from build123d import *

# Parameters (mm, degrees)
CYLINDER011007_R     = 2.1
CYLINDER011007_DEPTH = 20
CYLINDER011006_R     = 12
CYLINDER011006_DEPTH = 2
CYLINDER011009_R     = 0.5
CYLINDER011009_DEPTH = 7
ARRAY007_COUNT       = 22
CYLINDER011005_R     = 6
CYLINDER011005_DEPTH = 7


with BuildPart() as belt_attach_insert_hole:
    # Cylinder011007 → Cylinder011007 (new body)
    with BuildSketch(Plane.XZ):
        Circle(CYLINDER011007_R)
    extrude(amount=CYLINDER011007_DEPTH)


with BuildPart() as belt_disk:
    # Cylinder011006 → Cylinder011006 (new body)
    with BuildSketch(Plane.XZ.offset(7)):
        Circle(CYLINDER011006_R)
    extrude(amount=CYLINDER011006_DEPTH)


with BuildPart() as belt_pin_array:
    # Cylinder011009 → Cylinder011009 (new body)
    with BuildSketch(Plane(origin=(6, 0, 0), x_dir=(1, 0, 0), z_dir=(0, -1, 0))):
        Circle(CYLINDER011009_R)
    extrude(amount=CYLINDER011009_DEPTH)

    # Array007: belt pin array ×22 about axis
    array007_axis = Axis((0, 0, 0), (0, 1, 0))


with BuildPart() as belt_pin_array_1:
    add(belt_pin_array.part)
    for i in range(1, ARRAY007_COUNT):
        add(belt_pin_array.part.rotate(array007_axis, i * 360 / ARRAY007_COUNT))


with BuildPart() as belt_attach_cut:
    # Cylinder011005 → Cylinder011005 (new body)
    with BuildSketch(Plane.XZ):
        Circle(CYLINDER011005_R)
    extrude(amount=CYLINDER011005_DEPTH)

    # Fusion003: union belt disk, belt pin array
    add(belt_disk.part)
    add(belt_pin_array_1.part)

    # Cut023015009007: cut belt attach insert hole
    add(belt_attach_insert_hole.part, mode=Mode.SUBTRACT)


solid = belt_attach_cut.part
Geometry check sheet. Reference: the model listing, model coordinates, mm. A direction names the side the tool comes from. Coordinates: 2 decimals unless noted, no trailing zeros. Loops run counter-clockwise (first coordinate to the right, second up) from the corner with the lowest first, then second, coordinate; pieces in that order, holes last. Notation, with made-up numbers: (75, 34.25) - (123, 34.25) arc R35 cw to (123, 67.25) - close; hole circle Ø5 at (10, 77). An arc over 180 degrees is marked (long way). Use one line per item in the form item = value. Start each with the question number.
Item 1: Gauge pin test, flat ends, axial feed: pin 1 (4 mm diameter, centred on x = 0, z = 0, fed in from -Y); pin 2 (1 mm diameter, centred on x = 3.5, z = -6, fed in from +Y); pin 3 (4 mm diameter, centred on y = -5.5, z = 2.5, fed in from -X); pin 4 (5 mm diameter, centred on y = -1, z = -4.5, fed in from +X). Record the tip position at first contact, or that the pin passes through.
Item 2: Thickness scan on probe 1 along X at (y, z) = (-6, 0); probe 2 along Z at (x, y) = (0, -6.75); probe 3 along Z at (x, y) = (-2.5, -4.5). Record the ranges inside material, lowest first.
Item 3: Tool access check on faces 1 (the face through (2.003, -4.437, 0.631)), 2 (the face through (-6, -7, 3)). Record the directions out of +Z, -Z, +X, -X, +Y, -Y that give a thin tool (end or side, any length) a straight path to the whole face; none if there is none.
Item 4: Section check D-D, the plane x = -7. Enter the section's corners in (y, z), and give its area (3 significant figures).
Item 5: Section check B-B, the plane z = 0. Enter the section's corners in (x, y), and give its area (3 significant figures).
Item 6: Section check A-A, the plane x = 0. Enter the section's corners in (y, z).
Item 7: Section check C-C, the plane y = -8. Enter the section's corners in (x, z), and give its area (3 significant figures).
Item 8: Mould release check, pull along Z, two halves, no side actions. Record for faces 3 (the face through (2.5, -9, 0.2)), 4 (the face through (4.27, -3.45, 4.9)): +Z half, -Z half, draft (parallel to the pull), parting line (faces both ways), or undercut.
Computed:
q1.pin_1 = through
q1.pin_2 = -7
q1.pin_3 = -11.94
q1.pin_4 = 6.15
q2.probe_1 = -6.5 to -2.1, 2.1 to 6.5
q2.probe_2 = -6 to -2.1, 2.1 to 6
q2.probe_3 = -5.96 to 5.96
q3.face_1 = +Y, -Y
q3.face_2 = +Y
q4.outline = (-9, -9.75) - (-7, -9.75) - (-7, 9.75) - (-9, 9.75) - close
q4.area = 39.0 mm2
q5.outline = (-12, -9) - (-2.1, -9) - (-2.1, 0) - (-6.5, 0) - (-6.5, -7) - (-12, -7) - close; (2.1, -9) - (12, -9) - (12, -7) - (6.5, -7) - (6.5, 0) - (2.1, 0) - close
q5.area = 101 mm2
q6.outline = (-9, -12) - (-7, -12) - (-7, -6) - (0, -6) - (0, -2.1) - (-9, -2.1) - close; (-9, 2.1) - (0, 2.1) - (0, 6) - (-7, 6) - (-7, 12) - (-9, 12) - close
q7.outline = circle Ø24 at (0, 0); hole circle Ø4.2 at (0, 0)
q7.area = 439 mm2
q8.face_3 = draft
q8.face_4 = undercut
